```python
from build123d import *

# Parameters (mm, degrees)
BOSS_EXTRU_1_DEPTH = 3


with BuildPart() as part:
    # Esquisse1 → Boss.-Extru.1 (new body)
    with BuildSketch(Plane(origin=(3, 0, 0), x_dir=(0, 0, -1), z_dir=(1, 0, 0))):
        with BuildLine():
            Line((-5.105655505, -9.426547116), (-59.475655505, -9.426547116))
            Line((-59.475655505, -9.426547116), (-59.475655505, -42.788807913))
            ThreePointArc((-59.475655505, -42.788807913), (-26.377783326, -55.526547116), (-59.475655505, -68.264286319))
            Line((-59.475655505, -68.264286319), (-59.475655505, -78.526547116))
            Line((-59.475655505, -78.526547116), (-49.475655505, -78.526547116))
            Line((-49.475655505, -78.526547116), (-49.475655505, -81.526547116))
            Line((-49.475655505, -81.526547116), (-59.475655505, -81.526547116))
            Line((-59.475655505, -81.526547116), (-59.475655505, -106.426547116))
            Line((-59.475655505, -106.426547116), (-57.675655505, -106.426547116))
            Line((-57.675655505, -106.426547116), (-57.675655505, -109.426547116))
            Line((-57.675655505, -109.426547116), (-18.675655505, -109.426547116))
            Line((-18.675655505, -109.426547116), (-18.675655505, -106.426547116))
            Line((-18.675655505, -106.426547116), (-5.105655505, -106.426547116))
            Line((-5.105655505, -106.426547116), (-5.105655505, -9.426547116))
        make_face()
    extrude(amount=-BOSS_EXTRU_1_DEPTH)


solid = part.part
```
Verification items for the finished model (mm, model axes). A direction names the side the tool comes from. Round coordinates to 2 decimals unless told otherwise and drop trailing zeros. Order: outer loops, then holes, each group sorted by start corner. A loop starts at its lowest first (then second) coordinate and runs counter-clockwise, first axis right, second up. Notation, with made-up numbers: (-20.75, 19) -> (35.25, 19) arc R18 cw to (35.25, 46) -> close; hole circle Ø4 at (69, -7.5). An arc over 180 degrees is marked (long way). Put each result on its own line as item: value. Start each with the question number.
(1) Section check A-A (x = 0.85). Enter the section's corners in (y, z).
(2) Depth check by flat-ended pin: pin 1 Ø1.5 at (x, y) = (1.5, -107.5) entering from -Z; pin 2 Ø1.5 at (x, z) = (1.5, 17.5) entering from -Y. Enter the tip coordinate at first touch or a pass-through.
(3) Material ranges on line 1 along Y through (x, z) = (1.65, 53); line 2 along Y through (x, z) = (0.8, 45.5); line 3 along Y through (x, z) = (2.2, 54.5), recorded low to high.
(4) Section check B-B (y = -41). Enter the section's corners in (x, z).
(5) Draft check along Y on faces 1 (the face through (2, -109.427, 38)), 2 (the face through (2, -9.427, 32)), 3 (the face through (1.52, -54.89, 26.39)). Enter one of: +Y half, -Y half, draft (parallel to the pull), parting line (faces both ways), or undercut.
(6) Tool access check on faces 4 (the face through (2, -81.527, 54)), 5 (the face through (0, -59, 21)), 6 (the face through (2, -108, 57.676)), 7 (the face through (2, -106.427, 12)), 8 (the face through (2, -26, 59.476)). Record the directions out of +Z, -Z, +X, -X, +Y, -Y that give a thin tool (end or side, any length) a straight path to the whole face; none if there is none.
(7) Section check D-D (z = 12). Enter the section's corners in (x, y), then the cut area to 3 significant figures.
(8) Section check C-C (z = 33). Enter the section's corners in (x, y), then the cut area to 3 significant figures.
Completed:
1. outline: (-109.43, 18.68) -> (-106.43, 18.68) -> (-106.43, 5.11) -> (-9.43, 5.11) -> (-9.43, 59.48) -> (-42.79, 59.48) arc R19 cw (long way) to (-68.26, 59.48) -> (-78.53, 59.48) -> (-78.53, 49.48) -> (-81.53, 49.48) -> (-81.53, 59.48) -> (-106.43, 59.48) -> (-106.43, 57.68) -> (-109.43, 57.68) -> close
2. pin 1: stops at z = 18.68
2. pin 2: stops at y = -106.43
3. line 1: y = -109.43 to -81.53, -78.53 to -72.93, -38.12 to -9.43
3. line 2: y = -109.43 to -74.53, -36.53 to -9.43
3. line 3: y = -109.43 to -81.53, -78.53 to -72.19, -38.86 to -9.43
4. outline: (0, 5.11) -> (3, 5.11) -> (3, 33.13) -> (0, 33.13) -> close; (0, 57.62) -> (3, 57.62) -> (3, 59.48) -> (0, 59.48) -> close
5. face 1: -Y half
5. face 2: +Y half
5. face 3: undercut
6. face 4: +Z, +X, -X
6. face 5: +Z, -Z, -X, +Y, -Y
6. face 6: +Z, +X, -X, -Y
6. face 7: -Z, +X, -X, -Y
6. face 8: +Z, +X, -X, +Y, -Y
7. outline: (0, -106.43) -> (3, -106.43) -> (3, -9.43) -> (0, -9.43) -> close
7. area: 291 mm2
8. outline: (0, -109.43) -> (3, -109.43) -> (3, -69.94) -> (0, -69.94) -> close; (0, -41.11) -> (3, -41.11) -> (3, -9.43) -> (0, -9.43) -> close
8. area: 214 mm2
